from build123d import *

# Parameters (mm, degrees)
SKETCH1_R           = 15.875
SKETCH1_R_2         = 12.7
SKETCH1_W           = 73.66
SKETCH1_H           = 31.75
BOSS_EXTRUDE2_DEPTH = 6.35
CUT_EXTRUDE1_DEPTH  = 2.54
SKETCH3_R           = 4.7625
CUT_EXTRUDE2_DEPTH  = 7.35
CIRPATTERN1_COUNT   = 9


with BuildPart() as part:
    # Sketch1 → Boss-Extrude2 (new body)
    with BuildSketch(Plane(origin=(0, 0, 0), x_dir=(1, 0, 0), z_dir=(0, 1, 0))):
        with Locations((209.55, -47.625)):
            Circle(SKETCH1_R)
        with Locations((0, -57.15)):
            Circle(SKETCH1_R)
        with BuildLine():
            Line((209.55, -76.2), (209.55, -19.05))
            ThreePointArc((209.55, -19.05), (203.970384182, -5.579615818), (190.5, 0))
            Line((190.5, 0), (12.7, 0))
            Line((12.7, 0), (0, -12.7))
            Line((0, -12.7), (0, -101.6))
            ThreePointArc((0, -101.6), (35.56, -137.16), (71.12, -101.6))
            Line((71.12, -101.6), (71.12, -78.74))
            ThreePointArc((71.12, -78.74), (76.699615818, -65.269615818), (90.17, -59.69))
            Line((90.17, -59.69), (152.4, -59.69))
            ThreePointArc((152.4, -59.69), (156.890128061, -61.549871939), (158.75, -66.04))
            Line((158.75, -66.04), (158.75, -76.2))
            ThreePointArc((158.75, -76.2), (184.15, -101.6), (209.55, -76.2))
        make_face()
        with Locations((35.56, -101.6)):
            Circle(SKETCH1_R_2, mode=Mode.SUBTRACT)
        with Locations((184.15, -76.2)):
            Circle(SKETCH1_R, mode=Mode.SUBTRACT)
        with Locations((153.67, -26.035)):
            Rectangle(SKETCH1_W, SKETCH1_H, mode=Mode.SUBTRACT)
        with Locations((55.88, -26.035)):
            Rectangle(SKETCH1_W, SKETCH1_H, mode=Mode.SUBTRACT)
        with BuildLine():
            ThreePointArc((15.875, -57.15), (11.225320151, -45.924679849), (0, -41.275))
            Line((0, -41.275), (0, -73.025))
            ThreePointArc((0, -73.025), (11.225320151, -68.375320151), (15.875, -57.15))
        make_face()
        with BuildLine():
            Line((0, -73.025), (0, -41.275))
            ThreePointArc((0, -41.275), (-15.875, -57.15), (0, -73.025))
        make_face()
        with BuildLine():
            ThreePointArc((15.875, -57.15), (11.225320151, -45.924679849), (0, -41.275))
            Line((0, -41.275), (0, -73.025))
            ThreePointArc((0, -73.025), (11.225320151, -68.375320151), (15.875, -57.15))
        make_face()
        with BuildLine():
            Line((0, -73.025), (0, -41.275))
            ThreePointArc((0, -41.275), (-15.875, -57.15), (0, -73.025))
        make_face()
        with BuildLine():
            ThreePointArc((225.425, -47.625), (220.775320151, -36.399679849), (209.55, -31.75))
            Line((209.55, -31.75), (209.55, -63.5))
            ThreePointArc((209.55, -63.5), (220.775320151, -58.850320151), (225.425, -47.625))
        make_face()
        with BuildLine():
            Line((209.55, -63.5), (209.55, -31.75))
            ThreePointArc((209.55, -31.75), (193.675, -47.625), (209.55, -63.5))
        make_face()
        with BuildLine():
            ThreePointArc((225.425, -47.625), (220.775320151, -36.399679849), (209.55, -31.75))
            Line((209.55, -31.75), (209.55, -63.5))
            ThreePointArc((209.55, -63.5), (220.775320151, -58.850320151), (225.425, -47.625))
        make_face()
        with BuildLine():
            Line((209.55, -63.5), (209.55, -31.75))
            ThreePointArc((209.55, -31.75), (193.675, -47.625), (209.55, -63.5))
        make_face()
    extrude(amount=BOSS_EXTRUDE2_DEPTH)

    # Sketch2 → Cut-Extrude1 (cut)
    with BuildSketch(Plane(origin=(0, 6.35, 0), x_dir=(1, 0, 0), z_dir=(0, 1, 0))):
        with BuildLine():
            Line((209.55, -76.2), (209.55, -63.5))
            ThreePointArc((209.55, -63.5), (225.425, -47.625), (209.55, -31.75))
            Line((209.55, -31.75), (209.55, -19.05))
            ThreePointArc((209.55, -19.05), (203.970384182, -5.579615818), (190.5, 0))
            Line((190.5, 0), (12.7, 0))
            Line((12.7, 0), (0, -12.7))
            Line((0, -12.7), (0, -41.275))
            ThreePointArc((0, -41.275), (-15.875, -57.15), (0, -73.025))
            Line((0, -73.025), (0, -101.6))
            ThreePointArc((0, -101.6), (35.56, -137.16), (71.12, -101.6))
            Line((71.12, -101.6), (71.12, -78.74))
            ThreePointArc((71.12, -78.74), (76.699615818, -65.269615818), (90.17, -59.69))
            Line((90.17, -59.69), (152.4, -59.69))
            ThreePointArc((152.4, -59.69), (156.890128061, -61.549871939), (158.75, -66.04))
            Line((158.75, -66.04), (158.75, -76.2))
            ThreePointArc((158.75, -76.2), (184.15, -101.6), (209.55, -76.2))
        make_face()
        with BuildLine():
            Line((2.54, -13.752102448), (2.54, -44.059139639))
            ThreePointArc((2.54, -44.059139639), (-13.335, -57.15), (2.54, -70.240860361))
            Line((2.54, -70.240860361), (2.54, -101.6))
            ThreePointArc((2.54, -101.6), (35.56, -134.62), (68.58, -101.6))
            Line((68.58, -101.6), (68.58, -78.74))
            ThreePointArc((68.58, -78.74), (74.903564594, -63.473564594), (90.17, -57.15))
            Line((90.17, -57.15), (152.4, -57.15))
            ThreePointArc((152.4, -57.15), (158.686179285, -59.753820715), (161.29, -66.04))
            Line((161.29, -66.04), (161.29, -76.2))
            ThreePointArc((161.29, -76.2), (184.15, -99.06), (207.01, -76.2))
            Line((207.01, -76.2), (207.01, -60.715860361))
            ThreePointArc((207.01, -60.715860361), (222.885, -47.625), (207.01, -34.534139639))
            Line((207.01, -34.534139639), (207.01, -19.05))
            ThreePointArc((207.01, -19.05), (202.174332957, -7.375667043), (190.5, -2.54))
            Line((190.5, -2.54), (13.752102448, -2.54))
            Line((13.752102448, -2.54), (2.54, -13.752102448))
        make_face(mode=Mode.SUBTRACT)
    extrude(amount=-CUT_EXTRUDE1_DEPTH, mode=Mode.SUBTRACT)

    # Sketch3 → Cut-Extrude2 (cut, through all)
    with BuildSketch(Plane(origin=(0, 6.35, 0), x_dir=(1, 0, 0), z_dir=(0, 1, 0))):
        with Locations((35.56, -76.2)):
            Circle(SKETCH3_R)
    cut_extrude2 = extrude(amount=-CUT_EXTRUDE2_DEPTH, mode=Mode.SUBTRACT)

    # CirPattern1: Cut-Extrude2 ×9 about axis
    cirpattern1_axis = Axis((35.56, 0, 101.6), (0, 1, 0))
    for i in range(1, CIRPATTERN1_COUNT):
        add(cut_extrude2.rotate(cirpattern1_axis, i * 360 / CIRPATTERN1_COUNT), mode=Mode.SUBTRACT)


solid = part.part
Design review of the part built by this model. Coordinates are the model's own, in mm. A direction names the side the tool comes from. Coordinates: 2 decimals unless noted, no trailing zeros. Order: outer loops, then holes, each group sorted by start corner. A loop starts at its lowest first (then second) coordinate and runs counter-clockwise, first axis right, second up.
Item 1: Take a section at B-B, the plane x = 184.15. Write out the cut boundary in (y, z) (3 decimals).
Item 2: Take a section at A-A, the plane x = 35.56. Write out the cut boundary in (y, z), then the cut area to 3 significant figures.
Item 3: The part is to be moulded in two halves that separate along X. For faces 4 (the cylindrical face through (34.83, 5.1, 134.61)), 5 (the cylindrical face through (-15.87, 1.88, 56.8)), 6 (the cylindrical face through (76.55, 1.88, 65.42)), say which applies: pulls with the +X half, pulls with the -X half, needs draft (parallel to the pull), parting line crosses it, or undercut.
Item 4: For line 1 (Z direction, x = 35.56, y = 3); line 2 (Z direction, x = 184.15, y = 1.75) (3 decimals); line 3 (X direction, y = 3.5, z = 29.5), list the stretches that pass through material, from the lowest coordinate up.
Item 5: For pin 1 Ø3 at (y, z) = (1.5, 30.5) entering from -X; pin 2 Ø11 at (x, z) = (10.55, 97.19) entering from -Y; pin 3 Ø3 at (x, z) = (155.5, 72) entering from +Y; pin 4 Ø2 at (y, z) = (5.5, 82) entering from -X, all flat-tipped, find the tip position at first contact; note any pin that passes through.
Item 6: Take a section at C-C, the plane y = 2.75. Count the separate pieces of the cut face and the enclosed holes in it, then the cut area to 3 significant figures.
Item 7: For faces 1 (the flat face through (116.84, 3, 26)), 2 (the cylindrical face through (202.3, 5.1, 7.5)), 3 (the cylindrical face through (158.62, 5.1, 59.69)), list the 3-axis set-ups (+Z, -Z, +X, -X, +Y, -Y) from which the entire face can be reached by the end or side of a thin tool; tool diameter is ignored.
The answers:
1. outline: (0, 0) - (3.81, 0) - (3.81, 2.54) - (6.35, 2.54) - (6.35, 10.16) - (0, 10.16) - close; (0, 41.91) - (6.35, 41.91) - (6.35, 60.325) - (0, 60.325) - close; (0, 92.075) - (6.35, 92.075) - (6.35, 99.06) - (3.81, 99.06) - (3.81, 101.6) - (0, 101.6) - close
2. outline: (0, 0) - (3.81, 0) - (3.81, 2.54) - (6.35, 2.54) - (6.35, 10.16) - (0, 10.16) - close; (0, 41.91) - (6.35, 41.91) - (6.35, 71.44) - (0, 71.44) - close; (0, 80.96) - (6.35, 80.96) - (6.35, 88.9) - (0, 88.9) - close; (0, 114.3) - (6.35, 114.3) - (6.35, 134.62) - (3.81, 134.62) - (3.81, 137.16) - (0, 137.16) - close
2. area: 435 mm2
3. face 4: parting line crosses it
3. face 5: pulls with the -X half
3. face 6: undercut
4. line 1: z = 0 to 10.16, 41.91 to 71.44, 80.96 to 88.9, 114.3 to 137.16
4. line 2: z = 0 to 10.16, 41.91 to 60.325, 92.075 to 101.6
4. line 3: x = 0 to 19.05, 92.71 to 116.84, 190.5 to 209.55
5. pin 1: stops at x = 0
5. pin 2: stops at y = 0
5. pin 3: passes through
5. pin 4: stops at x = 2.54
6. separate pieces: 1
6. enclosed holes: 13
6. area: 13,400 mm2
7. face 1: +Y, -Y
7. face 2: -Z, +X, +Y
7. face 3: +Z, +Y
